The figure shows three views and two pictorial views of one solid part (mm, origin at its lowest corner). Answer the questions. Coordinates: 2 decimals unless noted, no trailing zeros. Order: outer loops, then holes, each group sorted by start corner. A loop starts at its lowest first (then second) coordinate and runs counter-clockwise, first axis right, second up. Notation, with made-up numbers: (-13, 42) -> (-6, 42) arc R20 ccw to (-6, 53) -> close; hole circle Ø11 at (-39, 82.5). An arc over 180 degrees is marked (long way). Use one line per item in the form item = value.
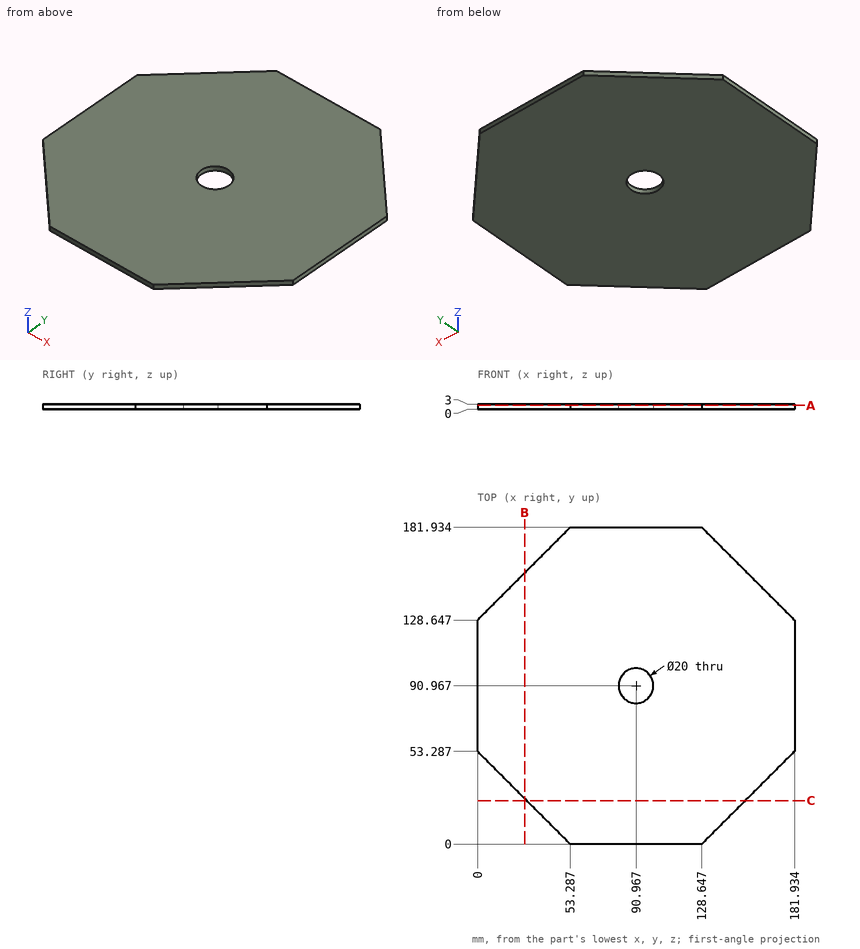
(1) Section C-C on y = 25 is taken. Write down the section's boundary in (x, z).
Data:
outline = (28.29, 0) -> (153.65, 0) -> (153.65, 3) -> (28.29, 3) -> close
(2) Section A-A on z = 2.2 is taken. Write down the section's boundary in (x, y), plus the area to 3 significant figures.
Data:
outline = (0, 53.29) -> (53.29, 0) -> (128.65, 0) -> (181.93, 53.29) -> (181.93, 128.65) -> (128.65, 181.93) -> (53.29, 181.93) -> (0, 128.65) -> close; hole circle Ø20 at (90.97, 90.97)
area = 27,100 mm²
(3) Straight lines are drawn through the part: line 1 along Y through (x, z) = (145.5, 2.45); line 2 along Y through (x, z) = (10, 2.6); line 3 along X through (y, z) = (82.5, 1.6) (1 decimal). For each, find the intervals that lie inside material, in ascending order.
Data:
line_1 = 16.85 to 165.08
line_2 = 43.29 to 138.65
line_3 = 0 to 85.6, 96.3 to 181.9
(4) Section B-B on x = 27 is taken. Write down the section's boundary in (y, z), plus the area to 3 significant figures.
Data:
outline = (26.29, 0) -> (155.65, 0) -> (155.65, 3) -> (26.29, 3) -> close
area = 388 mm²
